```python
from build123d import *

# Parameters (mm, degrees)
CROQUIS3_R              = 85
SALIENTE_EXTRUIR1_DEPTH = 3


with BuildPart() as part:
    # Croquis3 → Saliente-Extruir1 (new body)
    with BuildSketch(Plane(origin=(0, 0, 0), x_dir=(1, 0, 0), z_dir=(0, 1, 0))):
        with Locations(Location((0, 0, 0), (0, 0, 270))):
            Circle(CROQUIS3_R)
        with BuildLine():
            Line((-4.87398, 68.6), (-4.87398, 17.119705575))
            ThreePointArc((-4.87398, 17.119705575), (9.231788563, 15.218872492), (17.434798803, 3.587170289))
            Line((17.434798803, 3.587170289), (65.3213327, -24.060132946))
            Line((65.3213327, -24.060132946), (61.8463327, -30.079009502))
            Line((61.8463327, -30.079009502), (17.263089933, -4.33886229))
            ThreePointArc((17.263089933, -4.33886229), (8.564035914, -15.604399664), (-5.610818803, -16.892563818))
            Line((-5.610818803, -16.892563818), (-53.4973527, -44.539867054))
            Line((-53.4973527, -44.539867054), (-56.9723527, -38.520990498))
            Line((-56.9723527, -38.520990498), (-12.389109933, -12.780843285))
            ThreePointArc((-12.389109933, -12.780843285), (-17.795824477, 0.385527171), (-11.82398, 13.305393529))
            Line((-11.82398, 13.305393529), (-11.82398, 68.6))
            Line((-11.82398, 68.6), (-4.87398, 68.6))
        make_face(mode=Mode.SUBTRACT)
    extrude(amount=SALIENTE_EXTRUIR1_DEPTH)


solid = part.part
```
Design review of the part built by this model. Coordinates are the model's own, in mm. A direction names the side the tool comes from. Give positions to 0.01 mm unless a question says otherwise; leave off trailing zeros. Loops run counter-clockwise (first coordinate to the right, second up) from the corner with the lowest first, then second, coordinate; pieces in that order, holes last. Notation, with made-up numbers: M -34.75,53 L 14.25,53 A9 cw 14.25,64 Z; hole C 56.25,47.5 d6. An arc over 180 degrees is marked long. Return JSON: item names as keys, results as strings. Group by question number.
Item 1: Insertion check: pin 1 Ø4 at (x, z) = (45.5, -18) entering from -Y; pin 2 Ø1.5 at (y, z) = (1, -51.5) entering from -X; pin 3 Ø1.5 at (y, z) = (1, -30.5) entering from +X. Each pin has a flat end and moves straight along its axis. Give the tip position at first contact, or say it passes through.
Item 2: Tool access review of faces 1 (the flat face through (1, 0, -20)), 2 (the cylindrical face through (8.743, 1.479, 15.505)): name each direction out of +Z, -Z, +X, -X, +Y, -Y from which nothing blocks a thin tool from reaching the whole face with its end or side.
Item 3: We need section C-C (z = 0). Give the boundary of the cut face in (x, y), and give its area (3 significant figures).
Item 4: We need section B-B (x = 0). Give the boundary of the cut face in (y, z), and give its area (3 significant figures).
Item 5: For probe 1 along X at (y, z) = (1.8, 21); probe 2 along X at (y, z) = (0.55, -63); probe 3 along Z at (x, y) = (15, 0.5), list the stretches that pass through material, from the lowest coordinate up.
Item 6: We need section A-A (y = 1.8). Give the boundary of the cut face in (x, z), and give its area (3 significant figures).
Item 7: We need section D-D (z = 54.5). Give the boundary of the cut face in (x, y), and give its area (3 significant figures).
Item 8: Mouldability with a two-part tool opening along X and no side actions: class faces 3 (the cylindrical face through (-51.721, 1.479, -67.453)), 4 (the flat face through (-34.99, 1.48, 25.83)), 5 (the cylindrical face through (9.1, 1.5, -15.3)), 6 (the flat face through (1, 3, -20)) as released by +X, released by -X, zero draft, split by the parting line, or undercut.
Output:
{
 "1": {"pin 1": "stops at y = 0", "pin 2": "stops at x = -68.19", "pin 3": "stops at x = 79.62"},
 "2": {"face 1": "+Z, -Z, +X, -X, -Y", "face 2": "+Y, -Y"},
 "3": {"outline": "M -85,0 L -17.8,0 L -17.8,3 L -85,3 Z; M 23.65,0 L 85,0 L 85,3 L 23.65,3 Z", "area": "386 mm^2"},
 "4": {"outline": "M 0,-85 L 3,-85 L 3,-17.8 L 0,-17.8 Z; M 0,17.8 L 3,17.8 L 3,85 L 0,85 Z", "area": "403 mm^2"},
 "5": {"probe 1": "x = -82.37 to -26.63, -12.73 to 46.12, 60.02 to 82.37", "probe 2": "x = -57.06 to -11.82, -4.87 to 57.06", "probe 3": "z = -83.67 to -9.58, 9.58 to 83.67"},
 "6": {"outline": "C 0,0 d170; hole M -56.97,38.52 L -12.39,12.78 A17.8 ccw -11.82,-13.31 L -11.82,-68.6 L -4.87,-68.6 L -4.87,-17.12 A17.8 ccw 17.43,-3.59 L 65.32,24.06 L 61.85,30.08 L 17.26,4.34 A17.8 ccw -5.61,16.89 L -53.5,44.54 Z", "area": "20,600 mm^2"},
 "7": {"outline": "M -65.23,0 L 65.23,0 L 65.23,3 L -65.23,3 Z", "area": "391 mm^2"},
 "8": {"face 3": "split by the parting line", "face 4": "undercut", "face 5": "undercut", "face 6": "zero draft"}
}
